```python
from build123d import *

# Parameters (mm, degrees)
F0_W      = 64
F0_H      = 64
F1_DEPTH  = 2
F2_W      = 64
F2_H      = 2
F3_DEPTH  = 25
F4_W      = 64
F4_H      = 2
F5_DEPTH  = 90
F6_W      = 2
F6_H      = 92
F7_DEPTH  = 22
F8_W      = 2
F8_H      = 92
F9_DEPTH  = 22
F10_W     = 2
F10_H     = 92
F11_DEPTH = 60
F12_W     = 60
F12_H     = 2
F13_DEPTH = 20
F14_W     = 10
F14_H     = 20
F15_DEPTH = 25
F16_W     = 20
F16_H     = 20
F17_DEPTH = 25
F3_FACE_W = 64
F3_FACE_H = 2
F18_DEPTH = 15
F19_W     = 30
F19_H     = 2
F20_DEPTH = 2
F22_DEPTH = 40
F23_W     = 2
F23_H     = 24
F24_DEPTH = 5
F25_W     = 24
F25_H     = 2
F26_DEPTH = 2
F27_W     = 24
F27_H     = 2.5
F28_DEPTH = 2


with BuildPart() as f1:
    # F0 (on Top) → F1 (new body)
    with BuildSketch(Plane.XY):
        Rectangle(F0_W, F0_H)
    extrude(amount=F1_DEPTH)

    # F2 (on face) → F3 (join)
    with BuildSketch(Plane(origin=(0, 0, 0), x_dir=(1, 0, 0), z_dir=(0, 0, -1))):
        with Locations((0, 31)):
            Rectangle(F2_W, F2_H)
    extrude(amount=F3_DEPTH)

    # F4 (on face) → F5 (join)
    with BuildSketch(Plane(origin=(0, 0, 0), x_dir=(1, 0, 0), z_dir=(0, 0, -1))):
        with Locations((0, -31)):
            Rectangle(F4_W, F4_H)
    extrude(amount=F5_DEPTH)

    # F6 (on face) → F7 (join)
    with BuildSketch(Plane(origin=(0, 32, 0), x_dir=(-1, 0, 0), z_dir=(0, 1, 0))):
        with Locations((-31, -44)):
            Rectangle(F6_W, F6_H)
    extrude(amount=F7_DEPTH)

    # F8 (on face) → F9 (join)
    with BuildSketch(Plane(origin=(0, 32, 0), x_dir=(-1, 0, 0), z_dir=(0, 1, 0))):
        with Locations((31, -44)):
            Rectangle(F8_W, F8_H)
    extrude(amount=F9_DEPTH)

    # F10 (on face) → F11 (join)
    with BuildSketch(Plane(origin=(30, 0, 0), x_dir=(0, -1, 0), z_dir=(-1, 0, 0))):
        with Locations((-53, -44)):
            Rectangle(F10_W, F10_H)
    extrude(amount=F11_DEPTH)

    # F12 (on face) → F13 (join)
    with BuildSketch(Plane(origin=(0, 32, 0), x_dir=(-1, 0, 0), z_dir=(0, 1, 0))):
        with Locations((0, -89)):
            Rectangle(F12_W, F12_H)
    extrude(amount=F13_DEPTH)

    # F14 (on face) → F15 (cut)
    with BuildSketch(Plane.YZ.offset(32)):
        with Locations((37, -10)):
            Rectangle(F14_W, F14_H)
    extrude(amount=-F15_DEPTH, mode=Mode.SUBTRACT)

    # F16 (on face) → F17 (cut)
    with BuildSketch(Plane(origin=(0, 0, -90), x_dir=(1, 0, 0), z_dir=(0, 0, -1))):
        with Locations((-20, -42)):
            Rectangle(F16_W, F16_H)
    extrude(amount=-F17_DEPTH, mode=Mode.SUBTRACT)

    # F3_face (on face) → F18 (join)
    with BuildSketch(Plane(origin=(0, -31, -25), x_dir=(1, 0, 0), z_dir=(0, 0, -1))):
        Rectangle(F3_FACE_W, F3_FACE_H)
    extrude(amount=F18_DEPTH)

    # F19 (on face) → F20 (cut)
    with BuildSketch(Plane(origin=(0, 54, 0), x_dir=(-1, 0, 0), z_dir=(0, 1, 0))):
        with Locations((-15, -49)):
            Rectangle(F19_W, F19_H)
    extrude(amount=-F20_DEPTH, mode=Mode.SUBTRACT)

    # F21 (on face) → F22 (join)
    with BuildSketch(Plane.YZ.offset(32)):
        Polygon((30, 2), (30, 0), (32, 0), (42, 0), (54, 0), (54, 2), align=None)
    extrude(amount=F22_DEPTH)

    # F23 (on face) → F24 (join)
    with BuildSketch(Plane(origin=(0, 0, 0), x_dir=(1, 0, 0), z_dir=(0, 0, -1))):
        with Locations((71, -42)):
            Rectangle(F23_W, F23_H)
        Polygon((42, -54), (44, -54), (44, -47.911588), (44, -30), (42, -30), align=None)
    extrude(amount=F24_DEPTH)

    # F25 (on face) → F26 (join)
    with BuildSketch(Plane.YZ.offset(44)):
        with Locations((42, -4)):
            Rectangle(F25_W, F25_H)
    extrude(amount=F26_DEPTH)

    # F27 (on face) → F28 (join)
    with BuildSketch(Plane(origin=(70, 0, 0), x_dir=(0, -1, 0), z_dir=(-1, 0, 0))):
        with Locations((-42, -3.75)):
            Rectangle(F27_W, F27_H)
    extrude(amount=F28_DEPTH)


solid = f1.part
```
Geometry check sheet. Reference: the model listing, model coordinates, mm. A direction names the side the tool comes from. Coordinates: 2 decimals unless noted, no trailing zeros. Loops run counter-clockwise (first coordinate to the right, second up) from the corner with the lowest first, then second, coordinate; pieces in that order, holes last.
Item 1: Access from +Z, -Z, +X, -X, +Y, -Y to the whole of each face (thin tool, end or side, straight path). Record for faces 4 (the face through (52, 30, 1)), 5 (the face through (42, 42, -2)), 6 (the face through (-30, 42, -45)), 7 (the face through (70, 42, -1)), 8 (the face through (44, 42, -5)).
Item 2: Sectioned sample at C-C, the plane y = 37. Record the boundary of the cut face in (x, z).
Item 3: Thickness scan on line 1 (Y direction, x = 20, z = -18.5); line 2 (Y direction, x = 27, z = -41); line 3 (X direction, y = 41, z = -27). Record the ranges inside material, lowest first.
Item 4: Sectioned sample at A-A, the plane z = -36.5. Record the boundary of the cut face in (x, y).
Item 5: Release check for a two-part mould opening along X. For faces 1 (the face through (-2, 54, -45)), 2 (the face through (32, -15, 1)), 3 (the face through (68, 42, -4)) record: released by +X, released by -X, zero draft, split by the parting line, or undercut.
Item 6: Sectioned sample at B-B, the plane x = -26. Record the boundary of the cut face in (y, z), then the cut area to 3 significant figures.
Item 7: Go/stop test with flat-tipped pins: pin 1 Ø2 at (x, z) = (34, -78) entering from -Y (3 decimals); pin 2 Ø2 at (x, y) = (-1.5, -31) entering from -Z; pin 3 Ø22 at (y, z) = (45, -27.5) entering from +X; pin 4 Ø3.5 at (x, z) = (47, 0) entering from -Y. Record where each tip stops, or that it passes through.
Item 8: Sectioned sample at D-D, the plane z = -57.5. Record the boundary of the cut face in (x, y).
Check result:
1. face 4: +Z, -Z, +X, -Y
1. face 5: -Z, +Y, -Y
1. face 6: +Z, -Z
1. face 7: +Y, -Y
1. face 8: -Z, +X, +Y, -Y
2. outline: (-32, -90) - (-30, -90) - (-30, 2) - (-32, 2) - close; (-10, -90) - (32, -90) - (32, -20) - (30, -20) - (30, -88) - (-10, -88) - close; (30, 0) - (42, 0) - (42, -5) - (46, -5) - (46, -3) - (44, -3) - (44, 0) - (70, 0) - (70, -2.5) - (68, -2.5) - (68, -5) - (72, -5) - (72, 2) - (30, 2) - close
3. line 1: y = -32 to -30, 30 to 32, 52 to 54
3. line 2: y = 30 to 32, 52 to 54
3. line 3: x = -32 to -30, 30 to 32
4. outline: (-32, -32) - (32, -32) - (32, -30) - (-32, -30) - close; (-32, 30) - (32, 30) - (32, 54) - (-32, 54) - close; hole (-30, 32) - (30, 32) - (30, 52) - (-30, 52) - close
5. face 1: zero draft
5. face 2: released by +X
5. face 3: undercut
6. outline: (-32, -40) - (-30, -40) - (-30, 0) - (30, 0) - (30, -90) - (32, -90) - (32, 2) - (-32, 2) - close; (52, -90) - (54, -90) - (54, 2) - (52, 2) - close
6. area: 572 mm2
7. pin 1: passes through
7. pin 2: stops at z = -40
7. pin 3: stops at x = 32
7. pin 4: stops at y = 30
8. outline: (-32, 30) - (32, 30) - (32, 54) - (-32, 54) - close; hole (-30, 32) - (30, 32) - (30, 52) - (-30, 52) - close
